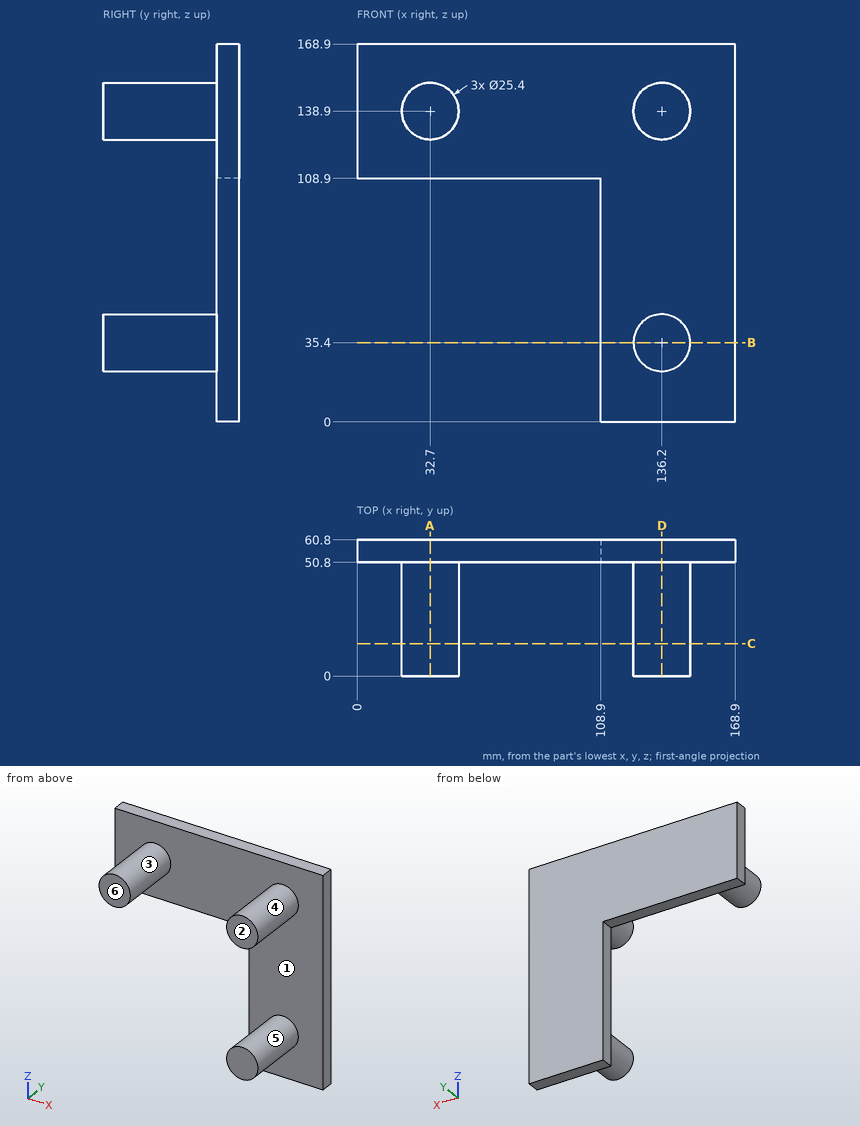
Input: dimensioned drawing with shaded views. Units: mm. Origin: part minimum x, y, z. A direction names the side the tool comes from. Coordinates: 2 decimals unless noted, no trailing zeros. Loops run counter-clockwise (first coordinate to the right, second up) from the corner with the lowest first, then second, coordinate; pieces in that order, holes last. Notation, with made-up numbers: M -24,-18.75 L -11,-18.75 A17 cw -11,-13.75 Z; hole C -11.5,67 d7. An arc over 180 degrees is marked long. One line per item, written item: value. Start each with the question number.
1) Draft query along X for the marked faces 3, 4, 5 and 6. Return one class per face: released by +X, released by -X, zero draft, split by the parting line, or undercut.
2) Reachability of the marked faces 1 and 2 from +Z, -Z, +X, -X, +Y, -Y: full face, straight path, thin tool, end or side. Return the list, or none.
3) Cut plane A-A (x = 32.7). Return loops of the section in (y, z).
4) Cut plane D-D (x = 136.2). Return loops of the section in (y, z), then the cut area to 3 significant figures.
5) Material intervals for L1, parallel to Y at x = 57, z = 117.5; L2, parallel to Z at x = 143, y = 47.5; L3, parallel to Z at x = 56, y = 55.5, sorted ascending. Write a range as from..to.
6) Cut plane C-C (y = 14.5). Return loops of the section in (x, z), then the cut area to 3 significant figures.
7) Pin query (flat end, axial travel): P1, Ø6, axis at x = 31.5, z = 112, coming from the -Y side; P2, Ø3, axis at x = 47.5, y = 56.5, coming from the -Z side; P3, Ø12, axis at x = 32.5, y = 14, coming from the -Z side. Return the tip coordinate at first contact, or that it passes through.
8) Cut plane B-B (z = 35.4). Return loops of the section in (x, y), then the cut area to 3 significant figures.
Evaluation:
1. face 3: undercut
1. face 4: undercut
1. face 5: split by the parting line
1. face 6: zero draft
2. face 1: -Y
2. face 2: +Z, -Z, +X, -X, -Y
3. outline: M 0,126.2 L 50.8,126.2 L 50.8,108.9 L 60.8,108.9 L 60.8,168.9 L 50.8,168.9 L 50.8,151.6 L 0,151.6 Z
4. outline: M 0,22.7 L 50.8,22.7 L 50.8,0 L 60.8,0 L 60.8,168.9 L 50.8,168.9 L 50.8,151.6 L 0,151.6 L 0,126.2 L 50.8,126.2 L 50.8,48.1 L 0,48.1 Z
4. area: 4,270 mm^2
5. L1: 50.8..60.8
5. L2: 24.67..46.13, 128.17..149.63
5. L3: 108.9..168.9
6. outline: C 32.7,138.9 d25.4; C 136.2,35.4 d25.4; C 136.2,138.9 d25.4
6. area: 1,520 mm^2
7. P1: y = 50.8
7. P2: z = 108.9
7. P3: z = 126.2
8. outline: M 108.9,50.8 L 123.5,50.8 L 123.5,0 L 148.9,0 L 148.9,50.8 L 168.9,50.8 L 168.9,60.8 L 108.9,60.8 Z
8. area: 1,890 mm^2
